Autodesk Inventor part; units mm, degrees
ref_plane "Work Plane1" through (29, 0, 0) normal (0, -1, 0) x (1, 0, 0)
ref_plane "YZ Plane" through (0, 0, 0) normal (1, 0, 0) x (0, 1, 0)
ref_plane "XZ Plane" through (0, 0, 0) normal (0, 1, 0) x (-1, 0, 0)
sketch "Sketch1" plane through (0, 0, 0) normal (0, 0, 1) x (1, 0, 0)
  line L0 (0.2879, 0) -> (12.7, 0)
  line L1 (12.7, 0) -> (12.7, 2.413)
  line L2 (12.7, 2.413) -> (2.0322, 2.413)
  line L3 (2.0322, 2.413) -> (0.0001, 2.413)
  line L4 (0.0001, 2.413) -> (0, 2.413)
  line L5 (0, 2.413) -> (0, 4.5847)
  line L6 (0, 4.5847) -> (-2.5654, 4.5847)
  line L7 (-2.5654, 4.5847) -> (-2.5654, 1.8624)
  line L8 (-2.5654, 1.8624) -> (-0.7874, 1.8624)
  line L9 (-0.7874, 1.8624) -> (0.2879, 0)
  line L10 (-5.6185, 0) -> (15.7531, 0)
  line L11 (0, -0.9169) -> (0, 5.5016)
  line L12 (2.0322, 2.413) -> (0, 2.413) construction
  dimension "d1" = 10.6678
  dimension "d2" = 2.0321
  dimension "d3" = 2.5654
  dimension "d4" = 1.778
  dimension "d5" = 60
  dimension "d6" = 4.826
  dimension "d7" = 4.826
  dimension "d8" = 3.7248
  dimension "d9" = 9.1694
  dimension "d26" = 12.7
revolve "Body" add sketch "Sketch1" angle 360 about axis through (0.2879, 0, 0) along (1, 0, 0) contours L9 L11 L3 L2 L1 L0 | L9 L8 L7 L6 L5 L11
sketch "Sketch2" plane through (-2.5654, 0, 0) normal (-1, 0, 0) x (0, 0, 1)
  circle A0 centre (0, 0) radius 1.8624
  line L0 (0, -6.4186) -> (0, 6.4186)
  line L1 (-6.4186, 0) -> (6.4186, 0)
  line L2 (1.8624, 0) -> (0.9312, -1.6129)
  line L3 (0.9312, -1.6129) -> (-0.9312, -1.6129)
  line L4 (-0.9312, -1.6129) -> (-1.8624, 0)
  line L5 (-1.8624, 0) -> (-0.9312, 1.6129)
  line L6 (-0.9312, 1.6129) -> (0.9312, 1.6129)
  line L7 (0.9312, 1.6129) -> (1.8624, 0)
extrude "Slot" add sketch "Sketch2" against normal up to next contours L7 A0 | A0 L2 | L6 L0 A0 | A0 L0 L3 | L0 L6 A0 | A0 L3 L0 | L4 A0 | A0 L5
fillet "Fillet1" radius 1.778 1 edges at (-2.5654, -4.5847, 0)
thread "Thread"
chamfer "Chamfer1" distance 0.6492 distance2 0.6492 1 edges at (12.7, -2.413, 0) measured on face at (12.7, -0.2852, -0.7521)
ref_plane "Work Plane1" through (29, 0, 0) normal (0, -1, 0) x (1, 0, 0)
fillet "Fillet2" radius 0.1 1 edges at (0.0001, -2.413, 0)
equation "\"d30\" = R"
equation "\"d17\" = RR"
equation "\"d13\" = GEL"
equation "\"d15\" = -0.5 * SPD + 0.5 * GD"
equation "\"d16\" = GUL"
equation "\"d1\" = GEL"
equation "\"d3\" = KOH"
equation "\"d4\" = INTI"
equation "\"d6\" = GD"
equation "\"d7\" = BDM"
equation "\"d8\" = 1.1547 * SW"
equation "\"d9\" = KOD"
equation "\"d26\" = NLG"
equation "\"GD\" = NND"
equation "\"NLG\" = 12.7"
equation "\"GEL\" = 10.6678"
equation "\"KOD\" = 9.1694"
equation "\"KOH\" = 2.5654"
equation "\"INTI\" = 1.778"
equation "\"GAL\" = 2.032"
equation "\"GUL\" = 0.64922"
equation "\"BDM\" = NND"
equation "\"SW\" = 3.2258"
equation "\"RR\" = 1.778"
equation "\"SPD\" = GD1"
equation "\"R\" = 0.1"
equation "\"KR\" = 5.4102"
equation "\"GD1\" = 3.52755"
equation "\"THREADDIA\" = 4.826"
equation "\"FAWI\" = 45deg"
equation "\"KOH1\" = 1.778"
equation "\"NND\" = 4.826"
equation "\"TOA\" = 30deg"
equation "\"E0\" = 1.155 * SW"
properties part number "Unbrako - 10 x 1/2" material "Steel, Mild"
Source: CAD feature listing. Evaluate the final solid. Frame: model axes, mm. A direction names the side the tool comes from. Round coordinates to 2 decimals unless told otherwise and drop trailing zeros. Write each loop counter-clockwise with the first axis right and the second up, starting at its lowest first coordinate (ties: lowest second). Pieces come first, ordered by that corner, then holes. Notation, with made-up numbers: M -27.75,86 L -9.75,86 A27 cw -9.75,114 Z; hole C 55.25,19 d2. An arc over 180 degrees is marked long. Answer as a JSON object with one key per item and string values. Group by question number.
(1) Section query B-B on x = 0.5. Output: boundary loops of the cut face in (y, z).
(2) Ray query, line 1 (X direction, y = 2.5, z = -0.25); line 2 (Y direction, x = -1.5, z = 1); line 3 (Z direction, x = -1.5, y = 1). Return the intervals inside material, ascending. Write a range as [from, to].
(3) First-contact query: pin 1 (0.9 mm diameter, centred on x = -2, z = 0, fed in from -Y); pin 2 (3 mm diameter, centred on x = 7.5, y = -1.5, fed in from -Z); pin 3 (1.5 mm diameter, centred on x = 3, z = -1.5, fed in from -Y). Flat tips, straight axial feed; report the tip coordinate or a pass-through.
(4) Reachability of faces 1 (the flat face through (-1.6, 0.8, 1.4)), 2 (the flat face through (-2.565, -2, 0)), 3 (the cylindrical face through (5.992, -1.915, 1.468)) from +Z, -Z, +X, -X, +Y, -Y: full face, straight path, thin tool, end or side. Return the list, or none.
(5) Section query A-A on x = -1.5. Output: boundary loops of the cut face in (y, z).
(6) Mould query, pull axis Z, two halves, no side actions, for faces 4 (the cylindrical face through (-0.4, -3.64, 2.79)), 5 (the flat face through (12.7, 0, 0)), 6 (the flat face through (-2, -1.613, 0)). Classes: +Z half, -Z half, draft (parallel to the pull), parting line (faces both ways), or undercut.
Computed values:
{
 "1": {"outline": "C 0,0 d4.83"},
 "2": {"line 1": "[-2.57, 0]", "line 2": "[-4.32, -1.49], [1.49, 4.32]", "line 3": "[-4.32, -1.29], [1.29, 4.32]"},
 "3": {"pin 1": "y = -4.41", "pin 2": "z = -2.41", "pin 3": "y = -2.29"},
 "4": {"face 1": "-X", "face 2": "+Z, -Z, -X, +Y, -Y", "face 3": "+X"},
 "5": {"outline": "C 0,0 d8.87; hole M -1.61,-0.93 L 0,-1.86 L 1.61,-0.93 L 1.61,0.93 L 0,1.86 L -1.61,0.93 Z"},
 "6": {"face 4": "parting line", "face 5": "draft", "face 6": "undercut"}
}
